Check sheet for the modelled part. Datum: model origin and axes. Units: mm. A direction names the side the tool comes from. Coordinates: 2 decimals unless noted, no trailing zeros. Loops run counter-clockwise (first coordinate to the right, second up) from the corner with the lowest first, then second, coordinate; pieces in that order, holes last. Notation, with made-up numbers: M 67.25,85.5 L 104.25,85.5 A29 ccw 104.25,109.5 Z; hole C 33.5,-11.5 d2. An arc over 180 degrees is marked long. Return JSON: item names as keys, results as strings.
from build123d import *

# Parameters (mm, degrees)
F1_DEPTH       = 42
F2_R           = 5.08
F3_R           = 1.27
F4_W           = 25
F4_H           = 3.175
F5_DEPTH       = 12.7
F7_DEPTH       = 33
F8_T1_DEPTH    = 45.7
F8_T3_DEPTH    = 43.656565316
F8_T5_DEPTH    = 41.6709689227
F9_W           = 6.35
F9_H           = 3.175
F10_DEPTH      = 12
F10_DEPTH_BACK = 30
F12_DEPTH      = 21
F12_DEPTH_BACK = 4
F13_R          = 1.27


# Not quite as in the source:
# - a fillet or chamfer that OpenCascade refuses, or shapes differently, is made with other operations: its cross-section is extruded or revolved along the edge and cut away or added


with BuildPart() as f1:
    # F0 (on Right) → F1 (new body)
    with BuildSketch(Plane.YZ):
        with BuildLine():
            Line((0, 0), (0, 67.502))
            Line((0, 67.502), (1.85, 67.502))
            ThreePointArc((1.85, 67.502), (6.35, 72.002), (10.85, 67.502))
            ThreePointArc((10.85, 67.502), (10.7816348886, 66.7205832005), (10.5786167935, 65.962909355))
            Line((10.5786167935, 65.962909355), (16.5456649355, 63.7910814449))
            Line((16.5456649355, 63.7910814449), (12.8715844298, 84.6278274207))
            Line((12.8715844298, 84.6278274207), (-34.925, 76.2))
            Line((-34.925, 76.2), (-34.925, 73.152))
            Line((-34.925, 73.152), (-9.525, 73.152))
            Line((-9.525, 73.152), (-9.525, 61.152))
            Line((-9.525, 61.152), (-34.925, 61.152))
            Line((-34.925, 61.152), (-34.925, 58.104))
            Line((-34.925, 58.104), (-9.525, 48.1738181818))
            Line((-9.525, 48.1738181818), (-9.525, 36.22870531))
            Line((-9.525, 36.22870531), (-34.925, 31.75))
            Line((-34.925, 31.75), (-34.925, 28.702))
            Line((-34.925, 28.702), (-9.525, 28.702))
            Line((-9.525, 28.702), (-9.525, 16.702))
            Line((-9.525, 16.702), (-34.925, 16.702))
            Line((-34.925, 16.702), (-34.925, 13.654))
            Line((-34.925, 13.654), (0, 0))
        make_face()
    extrude(amount=F1_DEPTH)

    # F2
    f2_edges = [f1.edges().sort_by_distance(p)[0] for p in [
        (21, 12.871584, 84.627827),
        (21, 0, 0),
    ]]
    fillet(f2_edges, radius=F2_R)

    # F3
    f3_edges = [f1.edges().sort_by_distance(p)[0] for p in [
        (21, 16.545665, 63.791081),
        (21, -9.525, 28.702),
        (21, -9.525, 48.173818),
        (21, -9.525, 73.152),
        (21, -9.525, 61.152),
        (21, -9.525, 16.702),
        (21, -34.925, 16.702),
        (21, -34.925, 13.654),
        (21, -34.925, 28.702),
        (21, -34.925, 61.152),
        (21, -34.925, 58.104),
        (21, -34.925, 31.75),
        (21, -34.925, 73.152),
        (21, -34.925, 76.2),
        (21, -9.525, 36.228705),
    ]]
    fillet(f3_edges, radius=F3_R)

    # F4 (on face) → F5 (join)
    with BuildSketch(Plane(origin=(0, 0, 0), x_dir=(-1, 0, 0), z_dir=(0, 1, 0))):
        with Locations((-17.5, 9.0279602963)):
            Rectangle(F4_W, F4_H)
    extrude(amount=F5_DEPTH)

    # F6 (on face) → F7 (cut)
    with BuildSketch(Plane.YZ.offset(42)):
        Polygon((0, 16.702), (0, 67.502), (-9.525, 67.502), (-9.525, 80.67870531), (-34.925, 80.67870531), (-34.925, 4.2203272727), (-10.795, 4.2203272727), (-10.795, 16.702), align=None)
    extrude(amount=-F7_DEPTH, mode=Mode.SUBTRACT)

    # F8: fillet of radius 5.08 on 5 edges, made by hand

    # F8_s2 → F8_t1 (cut)
    with BuildSketch(Plane.YZ.offset(9)):
        with BuildLine():
            ThreePointArc((-4.445, 67.502), (-8.0371024484, 68.9898975516), (-9.525, 72.582))
            Line((-9.525, 72.582), (-9.525, 67.502))
            Line((-9.525, 67.502), (-4.445, 67.502))
        make_face()
        with BuildLine():
            ThreePointArc((-5.715, 16.702), (-9.3071024484, 15.2141024484), (-10.795, 11.622))
            Line((-10.795, 11.622), (-10.795, 16.702))
            Line((-10.795, 16.702), (-5.715, 16.702))
        make_face()
        with BuildLine():
            ThreePointArc((-5.08, 16.702), (-1.4878975516, 15.2141024484), (0, 11.622))
            Line((0, 11.622), (0, 16.702))
            Line((0, 16.702), (-5.08, 16.702))
        make_face()
    extrude(amount=F8_T1_DEPTH, mode=Mode.SUBTRACT)

    # F8_s4 → F8_t3 (cut)
    with BuildSketch(Plane.YZ.offset(9)):
        with BuildLine():
            ThreePointArc((-5.3271327425, 81.4189025689), (-8.336505771, 79.6814402408), (-9.525, 76.4160791836))
            Line((-9.525, 76.4160791836), (-9.525, 80.67870531))
            Line((-9.525, 80.67870531), (-5.3271327425, 81.4189025689))
        make_face()
    extrude(amount=F8_T3_DEPTH, mode=Mode.SUBTRACT)

    # F8_s6 → F8_t5 (cut)
    with BuildSketch(Plane.YZ.offset(9)):
        with BuildLine():
            ThreePointArc((-10.795, 7.6887148418), (-9.9104077053, 4.8242857213), (-7.5647030762, 2.9574361003))
            Line((-7.5647030762, 2.9574361003), (-10.795, 4.2203272727))
            Line((-10.795, 4.2203272727), (-10.795, 7.6887148418))
        make_face()
    extrude(amount=F8_T5_DEPTH, mode=Mode.SUBTRACT)

    # F9 (on face) → F10 (join, two sides)
    with BuildSketch(Plane.YZ.offset(30)) as f10_sk:
        with Locations((9.525, 9.0279602963)):
            Rectangle(F9_W, F9_H)
    extrude(amount=F10_DEPTH)
    extrude(f10_sk.sketch, amount=-F10_DEPTH_BACK)

    # F11 (on face) → F12 (join, two sides)
    with BuildSketch(Plane.YZ.offset(9)) as f12_sk:
        Polygon((0, 57.502), (0, 67.502), (-3.175, 67.502), (-3.175, 54.327), (6.35, 54.327), (6.35, 57.502), align=None)
    extrude(amount=F12_DEPTH)
    extrude(f12_sk.sketch, amount=-F12_DEPTH_BACK)

    # F13
    f13_edges = [f1.edges().sort_by_distance(p)[0] for p in [
        (21, 12.7, 10.61546),
        (21, 12.7, 7.44046),
        (17.5, 6.35, 57.502),
        (17.5, 6.35, 54.327),
        (19.5, -3.175, 54.327),
    ]]
    fillet(f13_edges, radius=F13_R)


solid = f1.part
1) Scan lines: line 1 along Z through (x, y) = (11, 0.5); line 2 along Z through (x, y) = (28, 3.5); line 3 along Z through (x, y) = (5.5, -17). Record each from-to range of solid material in increasing order. Write a range as [from, to].
Answers:
{"line 1": "[7.44, 10.62], [54.33, 57.5], [67.5, 82.45]", "line 2": "[7.44, 10.62], [54.33, 57.5], [70.98, 82.98]", "line 3": "[6.65, 16.7], [28.7, 34.91], [51.1, 61.15], [73.15, 79.36]"}
2) Section check A-A on x = 32. Record the cut outline in (y, z) (3 decimals).
Answers:
{"outline": "M -10.795,7.689 A5.08 ccw -7.565,2.957 L -6.93,2.709 A5.08 ccw 0,7.44 L 0,11.622 A5.08 ccw -5.08,16.702 L -5.715,16.702 A5.08 ccw -10.795,11.622 Z; M -9.525,72.582 A5.08 ccw -4.445,67.502 L 1.85,67.502 A4.5 cw long 10.579,65.963 L 14.479,64.543 A1.27 ccw 16.164,65.957 L 13.754,79.625 A5.08 ccw 7.869,83.746 L -5.327,81.419 A5.08 ccw -9.525,76.416 Z; M 6.35,7.44 L 11.43,7.44 A1.27 ccw 12.7,8.71 L 12.7,9.345 A1.27 ccw 11.43,10.615 L 6.35,10.615 Z"}
3) Section check D-D on z = 33. Record the cut outline in (x, y).
Answers:
{"outline": "M 0,-27.84 L 9,-27.84 L 9,0 L 0,0 Z"}
4) Section check C-C on y = -31. Record the cut outline in (x, z).
Answers:
{"outline": "M 0,12.12 L 9,12.12 L 9,16.7 L 0,16.7 Z; M 0,28.7 L 9,28.7 L 9,32.44 L 0,32.44 Z; M 0,56.57 L 9,56.57 L 9,61.15 L 0,61.15 Z; M 0,73.15 L 9,73.15 L 9,76.89 L 0,76.89 Z"}
5) Go/stop test with flat-tipped pins: pin 1 Ø1.5 at (x, y) = (18, -10) entering from -Z; pin 2 Ø3.5 at (x, y) = (26, 3.5) entering from +Z; pin 3 Ø1 at (y, z) = (3.5, 9.5) entering from -X; pin 4 Ø8 at (x, z) = (36, 56) entering from +Y. Record where each tip stops, or that it passes through.
Answers:
{"pin 1": "z = 4.04", "pin 2": "z = 83.28", "pin 3": "x = 5", "pin 4": "through"}
6) Draft check along Y on faces 6 (the face through (0, -8, 43)), 7 (the face through (36, 6.35, 9)), 8 (the face through (25, -9.525, 75)), 9 (the face through (5, 3, 9)). Enter one of: +Y half, -Y half, draft (parallel to the pull), parting line (faces both ways), or undercut.
Answers:
{"face 6": "draft", "face 7": "undercut", "face 8": "-Y half", "face 9": "undercut"}
7) Set-up check for faces 1 (the face through (25, 1, 67.502)), 2 (the face through (18, 3, 57.502)), 3 (the face through (4, -22, 28.702)), 4 (the face through (25.27, -9.27, 15.25)), 5 (the face through (5, 3, 56)): record each of +Z, -Z, +X, -X, +Y, -Y from which the full face is reachable in a straight line by a thin tool's end or side.
Answers:
{"face 1": "+X", "face 2": "+X, -X, +Y", "face 3": "+X, -X, -Y", "face 4": "+X, -Y", "face 5": "-Z, -X, +Y"}
